Autodesk Inventor part; units mm, degrees
ref_plane "YZ Plane" through (0, 0, 0) normal (1, 0, 0) x (0, 1, 0)
ref_plane "XZ Plane" through (0, 0, 0) normal (0, 1, 0) x (-1, 0, 0)
ref_plane "XY Plane" through (0, 0, 0) normal (0, 0, 1) x (1, 0, 0)
sketch "Sketch1" plane through (0, 0, 0) normal (0, 0, 1) x (1, 0, 0)
  line L0 (-72.5, -44) -> (72.5, -44)
  line L1 (72.5, -44) -> (72.5, 44)
  line L2 (72.5, 44) -> (-72.5, 44)
  line L3 (-72.5, 44) -> (-72.5, -44)
  line L4 (-72.5, -44) -> (72.5, 44) construction
  line L5 (72.5, -44) -> (-72.5, 44) construction
  point P0 (0, 0)
  dimension "d0" = 145
  dimension "d1" = 88
extrude "Extrusion1" add sketch "Sketch1" along normal blind 7
sketch "Sketch2" plane through (0, 0, 7) normal (0, 0, 1) x (1, 0, 0)
  line L0 (-24.5465, 44) -> (-40.0633, -44) construction
  line L1 (18.9535, 44) -> (3.4367, -44) construction
  line L2 (72.5, 44) -> (-72.5, 44)
  line L3 (-72.5, -44) -> (72.5, -44)
  circle A0 centre (6.3902, -27.25) radius 1.75
  circle A1 centre (-27.5, 27.25) radius 1.75
  line L4 (-72.5, 44) -> (-72.5, -44)
  point P0 (0, 0)
  dimension "d4" = 80
  dimension "d5" = 43.5
  dimension "d6" = 3.5
  dimension "d7" = 3.5
  dimension "d8" = 54.5
  dimension "d9" = 16.75
  dimension "d10" = 88
  dimension "d11" = 45
sketch "Sketch3" plane through (0, 0, 0) normal (0, 0, -1) x (-1, 0, 0)
  line L0 (72.5, -44) -> (-72.5, -44)
  line L1 (-72.5, 44) -> (72.5, 44)
  line L2 (40, -44) -> (-60, -44)
  line L3 (-60, -44) -> (-60, 44)
  line L4 (-60, 44) -> (40, 44)
  line L5 (40, 44) -> (40, -44)
  line L6 (-72.5, -44) -> (-72.5, 44)
  line L7 (72.5, 44) -> (72.5, -44)
  point P0 (0, 0)
  point P1 (40, 44)
  point P2 (-60, -44)
  dimension "d14" = 100
  dimension "d15" = 145
  dimension "d16" = 32.5
extrude "Extrusion3" cut sketch "Sketch3" against normal blind 4 contours L0 L3 L1 L5
sketch "Sketch5" plane through (-72.5, -44, 7) normal (0, -1, 0) x (1, 0, 0)
  line L0 (145, -7) -> (132.5, -7)
  arc A0 (139, -7) -> (145, -4) centre (128.6677, 21.1646) ccw
  line L1 (145, -7) -> (145, 0)
  line L2 (132.5, -7) -> (145, -7)
  line L3 (132.5, -3) -> (132.5, -7)
  point P0 (72.5, -7)
  point P1 (132.5, -4)
  point P2 (139, -7)
  dimension "d25" = 4
  dimension "d26" = 6.5
  dimension "d27" = 30
extrude "Extrusion5" cut sketch "Sketch5" against normal through all
chamfer "Chamfer1" distance 0.5 angle 45 4 edges at (-72.5, 0, 7) (0, 44, 7) (72.5, 0, 7) (0, -44, 7)
sketch "Sketch7" plane through (0, 0, 4) normal (0, 0, -1) x (-1, 0, 0)
  line L0 (72.5, -44) -> (40, -44)
  line L1 (40, 44) -> (72.5, 44)
  line L2 (40, -44) -> (-60, -44)
  line L3 (40, -44) -> (40, 44)
  line L4 (40, -44) -> (47, -44)
  line L5 (47, -44) -> (41, 44)
  line L6 (41, 44) -> (40, 44)
  point P0 (0, 0)
  dimension "d34" = 7
  dimension "d35" = 1
extrude "Extrusion6" cut sketch "Sketch7" along normal through all
sketch "Sketch8" plane through (60, -44, 0) normal (0, -1, 0) x (1, 0, 0)
  point P0 (-60, 0)
ref_plane "Work Plane1" through (-47, -44, 2) normal (0.068, 0.9977, 0) x (0, 0, 1)
sketch "Sketch9" plane through (-47, -44, 2) normal (0.068, 0.9977, 0) x (0, 0, 1)
  line L0 (2, 0) -> (2, 106.7522)
  line L1 (2, 0) -> (-1, 20) construction
  line L2 (-1, 20) -> (-1, 54) construction
  line L3 (2, 106.7522) -> (2, 100.7661)
  line L4 (-1, 54) -> (2, 106.7522) construction
  spline S0 degree 3 poles (2, 0) (-1, 20) (-1, 54) (2, 106.7522) knots 1 1 1 1 2 2 2 2
  point P0 (-2, 43.8981)
equation "\"d9\" = -0.5 * d8 + 0.5 * d10"
properties part number "_3DPrint"
CAD build for the part. Positions are in the model's coordinates, mm. A direction names the side the tool comes from. Round coordinates to 2 decimals unless told otherwise and drop trailing zeros. Order: outer loops, then holes, each group sorted by start corner. A loop starts at its lowest first (then second) coordinate and runs counter-clockwise, first axis right, second up. Notation, with made-up numbers: (69.5, -27.5) - (115.5, -27.5) arc R24 cw to (115.5, 2.5) - close; hole circle Ø2 at (4.5, 28.5). An arc over 180 degrees is marked (long way). Use CSV: the item, a comma, the result in double quotes. Start each with the question number.
1) Tool access for faces 1 (the flat face through (-44.042, -0.616, 2.028)), 2 (the flat face through (-57, 1, 0)): list every direction of +Z, -Z, +X, -X, +Y, -Y with a clear straight run to the whole face (end or side of a thin tool).
2) Saw through at C-C (y = -20). List the corners of the cut face in (x, z).
3) Pin check, flat tip, straight feed: pin 1 Ø4 at (x, z) = (53.5, 1) entering from -Y. Stop position of the tip, or through.
4) Wall check: L1, parallel to X at y = 7, z = 3.75; L2, parallel to Z at x = 4.5, y = 28; L3, parallel to X at y = -2, z = 2.5. Give the ranges that are in metal, low to high. Write a range as [from, to].
5) Two-plate mould, pull along X, no slides. Class faces 3 (the flat face through (60, -1, 2)), 4 (the flat face through (72.5, -1, 5)), 5 (the flat face through (63, 1, 0)): pulls with the +X half, pulls with the -X half, needs draft (parallel to the pull), parting line crosses it, or undercut.
6) Saw through at B-B (x = 30.5). List the corners of the cut face in (y, z).
7) Saw through at A-A (y = -11). List the corners of the cut face in (x, z).
Values follow:
1,face 1,"-Z, -Y"
1,face 2,"-Z, +X, -X, +Y, -Y"
2,outline,"(-72.5, 0) - (-45.36, 0) - (-45.36, 4) - (60, 4) - (60, 0) - (66.5, 0) arc R30 ccw to (72.5, 3) - (72.5, 6.5) - (72, 7) - (-72, 7) - (-72.5, 6.5) - close"
3,pin 1,"passes through"
4,L1,"x = [-72.5, -43.52], [60, 72.5]"
4,L2,"z = [4, 7]"
4,L3,"x = [-72.5, -44.14], [60, 71.7]"
5,face 3,"undercut"
5,face 4,"pulls with the +X half"
5,face 5,"needs draft"
6,outline,"(-44, 4) - (44, 4) - (44, 6.5) - (43.5, 7) - (-43.5, 7) - (-44, 6.5) - close"
7,outline,"(-72.5, 0) - (-44.75, 0) - (-44.75, 4) - (60, 4) - (60, 0) - (66.5, 0) arc R30 ccw to (72.5, 3) - (72.5, 6.5) - (72, 7) - (-72, 7) - (-72.5, 6.5) - close"
